Here's how the part is built. I have some questions about the finished solid (model axes, mm). A direction names the side the tool comes from. Give positions to 0.01 mm unless a question says otherwise; leave off trailing zeros. Write each loop counter-clockwise with the first axis right and the second up, starting at its lowest first coordinate (ties: lowest second). Pieces come first, ordered by that corner, then holes. Notation, with made-up numbers: (48.25, 52.5) -> (76.25, 52.5) arc R7 cw to (76.25, 61.5) -> close; hole circle Ø5 at (-31.75, 6). An arc over 180 degrees is marked (long way). Put each result on its own line as item: value. Start each with the question number.
from build123d import *

# Parameters (mm, degrees)
F1_DEPTH = 4
F3_DEPTH = 16
F4_DEPTH = 25
F5_DEPTH = 25


with BuildPart() as f1:
    # F0 (on Top) → F1 (new body, symmetric)
    with BuildSketch(Plane.XY):
        Polygon((9.9233569652, 60.4344099144), (9.9233569652, 44.4344099144), (13.9233569652, 44.4344099144), (21.9233569652, 44.4344099144), (25.9233569652, 44.4344099144), (25.9233569652, 60.4344099144), align=None)
        with BuildLine():
            Line((9.9233569652, 4.4344099144), (12.4728915006, 0))
            Line((12.4728915006, 0), (16.0660725096, 3.580218208))
            ThreePointArc((16.0660725096, 3.580218208), (16.1752710503, 4.1253341753), (15.7131585893, 4.4344099144))
            Line((15.7131585893, 4.4344099144), (13.9233569652, 4.4344099144))
            Line((13.9233569652, 4.4344099144), (13.9233569652, 44.4344099144))
            Line((13.9233569652, 44.4344099144), (9.9233569652, 44.4344099144))
            Line((9.9233569652, 44.4344099144), (9.9233569652, 4.4344099144))
        make_face()
        with BuildLine():
            Line((25.9233569652, 44.4344099144), (21.9233569652, 44.4344099144))
            Line((21.9233569652, 44.4344099144), (21.9233569652, 4.4344099144))
            Line((21.9233569652, 4.4344099144), (20.1335553411, 4.4344099144))
            ThreePointArc((20.1335553411, 4.4344099144), (19.6714428801, 4.1253341753), (19.7806414208, 3.580218208))
            Line((19.7806414208, 3.580218208), (23.3738224298, 0))
            Line((23.3738224298, 0), (25.9233569652, 4.4344099144))
            Line((25.9233569652, 4.4344099144), (25.9233569652, 44.4344099144))
        make_face()
    extrude(amount=F1_DEPTH, both=True)

    # F2 (on face) → F3 (join, through all)
    with BuildSketch(Plane.YZ.offset(25.9233569652)):
        with BuildLine():
            Line((59.3626131447, -4), (52.4344099144, -4))
            Line((52.4344099144, -4), (45.5062066841, -4))
            ThreePointArc((45.5062066841, -4), (48.4344099144, -6.9282032303), (52.4344099144, -8))
            ThreePointArc((52.4344099144, -8), (56.4344099144, -6.9282032303), (59.3626131447, -4))
        make_face()
        with BuildLine():
            ThreePointArc((52.4344099144, -8), (48.4344099144, -6.9282032303), (45.5062066841, -4))
            Line((45.5062066841, -4), (4.4344099144, -4))
            Line((4.4344099144, -4), (0, -4))
            Line((0, -4), (0, -8))
            Line((0, -8), (52.4344099144, -8))
        make_face()
        with BuildLine():
            Line((45.5062066841, 4), (52.4344099144, 4))
            Line((52.4344099144, 4), (59.3626131447, 4))
            ThreePointArc((59.3626131447, 4), (52.4344099144, 8), (45.5062066841, 4))
        make_face()
    extrude(amount=-F3_DEPTH)

    # F2 (on face) → F4 (cut)
    with BuildSketch(Plane.YZ.offset(25.9233569652)):
        with BuildLine():
            ThreePointArc((52.4344099144, -4), (55.2628370391, -2.8284271247), (56.4344099144, 0))
            ThreePointArc((56.4344099144, 0), (55.2628370391, 2.8284271247), (52.4344099144, 4))
            ThreePointArc((52.4344099144, 4), (48.4344099144, 0), (52.4344099144, -4))
        make_face()
    extrude(amount=-F4_DEPTH, mode=Mode.SUBTRACT)

    # F5 (cut): faces of the model
    f5_faces = [f1.faces().sort_by_distance(p)[0] for p in [
        (17.9233569652, 22.5369531537, -4),
        (10.7732018103, 1.4781366381, -4),
        (25.0735121201, 1.4781366381, -4),
    ]]
    extrude(f5_faces, amount=-F5_DEPTH, mode=Mode.SUBTRACT)


solid = f1.part
1) I want a section at A-A, the plane y = 5.5. Write out the boundary of the cut face in (x, z).
2) I want a section at D-D, the plane z = 1.75. Write out the boundary of the cut face in (x, y), and give its area (3 significant figures).
3) I want a section at B-B, the plane z = -0.75. Write out the boundary of the cut face in (x, y), and give its area (3 significant figures).
4) I need wall thicknesses on probe 1 along Y at (x, z) = (14, -3.25); probe 2 along X at (y, z) = (36.5, -3.75); probe 3 along Y at (x, z) = (25.25, -3.5). Which ranges of each line are inside material? Lowest first, please.
5) I want a section at C-C, the plane x = 13.25. Write out the boundary of the cut face in (y, z).
6) I'm going to push flat-ended pins straight in: pin 1 Ø4 at (x, z) = (16.5, 0) entering from -Y; pin 2 Ø1.2 at (x, y) = (14.5, 60) entering from +Z; pin 3 Ø5 at (y, z) = (14.5, 5) entering from -X; pin 4 Ø0.5 at (x, y) = (16.5, 60) entering from -Z. Where does each tip first touch, or does it pass through?
7) Thinking about a two-plate mould opening in X: for faces 1 (the flat face through (18, 60, -4)), 2 (the flat face through (21.55, 1.82, -1.92)), 3 (the flat face through (9.923, 32, -2)), which applies, released by +X, released by -X, zero draft, split by the parting line, or undercut?
8) Which directions (+Z, -Z, +X, -X, +Y, -Y) give clear straight access to the entire face, cutting with the end or side of a thin tool? Please do faces 4 (the flat face through (23, 23, 4)), 5 (the flat face through (21.923, 25, -2)), 6 (the flat face through (24.631, 2.186, -1.916)), 7 (the flat face through (14.244, 1.765, -1.916)), 8 (the flat face through (18, 60, 4)).
Established:
1. outline: (9.92, -8) -> (13.92, -8) -> (13.92, 4) -> (9.92, 4) -> close; (21.92, -8) -> (25.92, -8) -> (25.92, 4) -> (21.92, 4) -> close
2. outline: (9.92, 4.43) -> (12.47, 0) -> (16.07, 3.58) arc R0.5 ccw to (15.71, 4.43) -> (13.92, 4.43) -> (13.92, 44.43) -> (21.92, 44.43) -> (21.92, 4.43) -> (20.13, 4.43) arc R0.5 ccw to (19.78, 3.58) -> (23.37, 0) -> (25.92, 4.43) -> (25.92, 48.84) -> (9.92, 48.84) -> close; (9.92, 56.03) -> (25.92, 56.03) -> (25.92, 60.43) -> (9.92, 60.43) -> close
2. area: 491 mm2
3. outline: (9.92, 4.43) -> (12.47, 0) -> (16.07, 3.58) arc R0.5 ccw to (15.71, 4.43) -> (13.92, 4.43) -> (13.92, 44.43) -> (21.92, 44.43) -> (21.92, 4.43) -> (20.13, 4.43) arc R0.5 ccw to (19.78, 3.58) -> (23.37, 0) -> (25.92, 4.43) -> (25.92, 48.51) -> (9.92, 48.51) -> close; (9.92, 56.36) -> (25.92, 56.36) -> (25.92, 60.43) -> (9.92, 60.43) -> close
3. area: 481 mm2
4. probe 1: y = 1.52 to 4.43, 44.43 to 50.1, 54.77 to 60.43
4. probe 2: x = 9.92 to 13.92, 21.92 to 25.92
4. probe 3: y = 3.26 to 50.5, 54.37 to 60.43
5. outline: (0.77, -8) -> (52.43, -8) arc R8 ccw to (59.36, -4) -> (60.43, -4) -> (60.43, 4) -> (59.36, 4) arc R8 ccw to (45.51, 4) -> (0.77, 4) -> close; hole circle Ø8 at (52.43, 0)
6. pin 1: stops at y = 2.02
6. pin 2: stops at z = 4
6. pin 3: stops at x = 9.92
6. pin 4: stops at z = -4
7. face 1: zero draft
7. face 2: undercut
7. face 3: released by -X
8. face 4: +Z, +X, -X, -Y
8. face 5: +Z, -Z
8. face 6: +Z, -Z, +X, -Y
8. face 7: +Z, -Z, -Y
8. face 8: +Z, +X, -X, +Y
